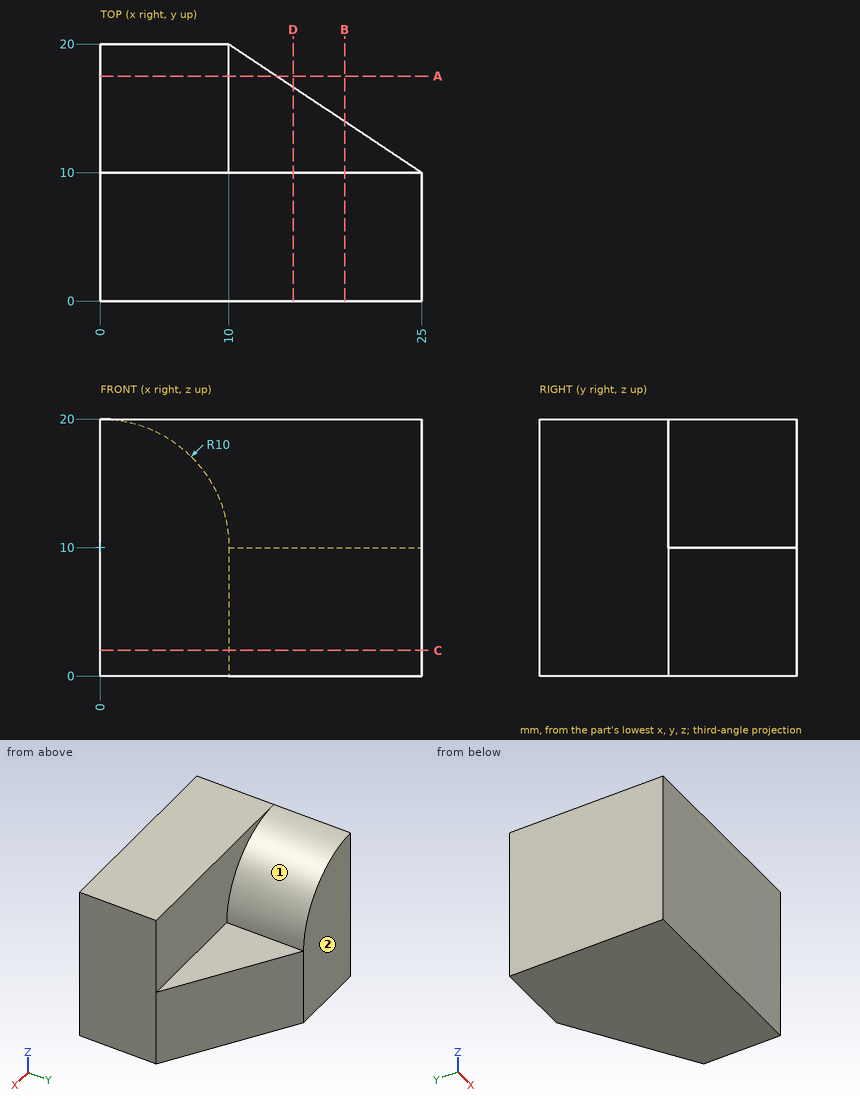
Can you work these out from the drawing? Everything is in mm from the part's minimum corner. A direction names the side the tool comes from. Round coordinates to 2 decimals unless told otherwise and drop trailing zeros. Loops run counter-clockwise (first coordinate to the right, second up) from the corner with the lowest first, then second, coordinate; pieces in that order, holes last. Notation, with made-up numbers: (-26.5, 76) - (29.5, 76) arc R20 cw to (29.5, 98) - close; hole circle Ø5 at (-34, -39). An arc over 180 degrees is marked (long way). One line per question, with ' | ' between items. Start each with the question number.
Q1. Will this pin go through, and if not, where does the flat tip stop? pin 1 (1.5 mm diameter, centred on x = 17.5, z = 13, fed in from +Y).
Q2. I want a section at A-A (y = 17.5). Write out the boundary of the cut face in (x, z).
Q3. I want a section at B-B (x = 19). Write out the boundary of the cut face in (y, z).
Q4. I want a section at C-C (z = 2). Write out the boundary of the cut face in (x, y), then the cut area to 3 significant figures.
Q5. I want a section at D-D (x = 15). Write out the boundary of the cut face in (y, z).
Q6. Please list where these lines run through material, in increasing order: line 1 (Z direction, x = 22, y = 11.25); line 2 (Z direction, x = 4, y = 15); line 3 (Y direction, x = 24, z = 9.25). Write a range as [from, to].
Q7. For the marked faces 1 and 2, which set-ups out of +Z, -Z, +X, -X, +Y, -Y let a thin tool reach every point of the face, with its end or its side?
Response values:
1) pin 1: stops at y = 10
2) outline: (0, 0) - (13.75, 0) - (13.75, 10) - (10, 10) arc R10 ccw to (0, 20) - close
3) outline: (0, 0) - (14, 0) - (14, 10) - (10, 10) - (10, 20) - (0, 20) - close
4) outline: (0, 0) - (25, 0) - (25, 10) - (10, 20) - (0, 20) - close | area: 425 mm²
5) outline: (0, 0) - (16.67, 0) - (16.67, 10) - (10, 10) - (10, 20) - (0, 20) - close
6) line 1: z = [0, 10] | line 2: z = [0, 19.17] | line 3: y = [0, 10.67]
7) face 1: +Z, +X, +Y | face 2: +Z, -Z, +X, -X, +Y
